The listing builds one solid part. Answer for the finished solid, in the listing's coordinates (mm). A direction names the side the tool comes from. Give positions to 0.01 mm unless a question says otherwise; leave off trailing zeros. Write each loop counter-clockwise with the first axis right and the second up, starting at its lowest first coordinate (ties: lowest second). Pieces come first, ordered by that corner, then holes. Notation, with made-up numbers: (80.5, -15) - (93.5, -15) arc R21 cw to (93.5, 23) - close; hole circle Ø6 at (60.5, 88.25). An arc over 180 degrees is marked (long way). One line per item, written item: value. Start each with the question number.
from build123d import *

# Parameters (mm, degrees)
F0_W     = 38.1
F0_H     = 88.9
F1_DEPTH = 76.2
F2_W     = 76.2
F2_H     = 152.4
F3_DEPTH = 317.5


# Not quite as in the source:
# - a feature names something its author has since deleted; it is built from what else it names


with BuildPart() as f1:
    # F0 (on Front) → F1 (new body, symmetric)
    with BuildSketch(Plane.XZ):
        Polygon((6.35, 1111.25), (-76.2, 1111.25), (-76.2, -1200.15), (76.2, -1200.15), (76.2, 1111.25), (44.45, 1111.25), align=None)
        with Locations((25.4, 1155.7)):
            Rectangle(F0_W, F0_H)
    extrude(amount=F1_DEPTH, both=True)

    # F2 (on face) → F3 (join)
    with BuildSketch(Plane(origin=(0, 0, -1200.15), x_dir=(1, 0, 0), z_dir=(0, 0, -1))):
        Rectangle(F2_W, F2_H)
    extrude(amount=F3_DEPTH)


solid = f1.part
Item 1: Find section A-A on y = 49. Determine the outline of the cut face in (x, z), plus the area to 3 significant figures.
Item 2: This flat-tipped pin is pushed along its axis until it touches: pin 1 Ø1 at (x, y) = (59, 11.5) entering from +Z. Where does it stop, or does it pass through?
Item 3: Straight lines are drawn through the part: line 1 along Z through (x, y) = (5.5, -59); line 2 along X through (y, z) = (-58.5, -1370.5); line 3 along Z through (x, y) = (-41.5, -68.5). For each, find the intervals that lie inside material, in ascending order.
Item 4: For faces 1 (the flat face through (-76.2, -1, -28)), 2 (the flat face through (-34, -1, 1111.25)), 3 (the flat face through (44.45, -1, 1155)), 4 (the flat face through (-38.1, 1, -1357)), 5 (the flat face through (38.1, 1, -1357)), determine the directions among +Z, -Z, +X, -X, +Y, -Y from which every point of the face is accessible in a straight line to the end or side of a thin tool.
Values:
1. outline: (-76.2, -1200.15) - (-38.1, -1200.15) - (-38.1, -1517.65) - (38.1, -1517.65) - (38.1, -1200.15) - (76.2, -1200.15) - (76.2, 1111.25) - (44.45, 1111.25) - (44.45, 1200.15) - (6.35, 1200.15) - (6.35, 1111.25) - (-76.2, 1111.25) - close
1. area: 380,000 mm^2
2. pin 1: z = 1111.25
3. line 1: -1517.65 to 1111.25
3. line 2: -38.1 to 38.1
3. line 3: -1200.15 to 1111.25
4. face 1: +Z, -Z, -X, +Y, -Y
4. face 2: +Z, -X, +Y, -Y
4. face 3: +Z, +X, +Y, -Y
4. face 4: -Z, -X, +Y, -Y
4. face 5: -Z, +X, +Y, -Y
